from build123d import *

# Parameters (mm, degrees)
F0_W     = 250
F0_H     = 300
F0_W_2   = 105
F0_H_2   = 135
F1_DEPTH = 100
F3_DEPTH = 297


with BuildPart() as f1:
    # F0 (on Front) → F1 (new body)
    with BuildSketch(Plane.XZ):
        with Locations((62.479706, 83.388156)):
            Rectangle(F0_W, F0_H)
        with Locations((62.479706, 83.388156)):
            Rectangle(F0_W_2, F0_H_2, mode=Mode.SUBTRACT)
    extrude(amount=F1_DEPTH)

    # F2 (on face) → F3 (cut)
    with BuildSketch(Plane.YZ.offset(187.479706)):
        Polygon((-30.774537, -66.611844), (-100, 233.388156), (-100, -66.611844), align=None)
    extrude(amount=-F3_DEPTH, mode=Mode.SUBTRACT)


solid = f1.part
Work out the finished part from the listing and answer in its coordinate system (mm). A direction names the side the tool comes from. Give positions to 0.01 mm unless a question says otherwise; leave off trailing zeros. Loops run counter-clockwise (first coordinate to the right, second up) from the corner with the lowest first, then second, coordinate; pieces in that order, holes last. Notation, with made-up numbers: M -30,-12 L 21,-12 A26 cw 21,6 Z; hole C -37.75,9.25 d9. An arc over 180 degrees is marked long. Use CSV: the item, a comma, the result in double quotes.
1) Find section B-B on x = 26. Write down the section's boundary in (y, z), plus the area to 3 significant figures.
Answer:
outline,"M -100,233.39 L -80.96,150.89 L 0,150.89 L 0,233.39 Z; M -49.81,15.89 L -30.77,-66.61 L 0,-66.61 L 0,15.89 Z"
area,"10,800 mm^2"
2) Find section C-C on z = 94. Write down the section's boundary in (x, y), plus the area to 3 significant figures.
Answer:
outline,"M -62.52,-67.84 L 9.98,-67.84 L 9.98,0 L -62.52,0 Z; M 114.98,-67.84 L 187.48,-67.84 L 187.48,0 L 114.98,0 Z"
area,"9,840 mm^2"
3) Determine the mould class of faces 3 (the flat face through (-62.52, -38, 115)), 4 (the flat face through (119.785, -64.903, 81.288)), 5 (the flat face through (114.98, -31, 82)), 6 (the flat face through (62, -25, 15.888)) for opening direction X: released by +X, released by -X, zero draft, split by the parting line, or undercut.
Answer:
face 3,"released by -X"
face 4,"zero draft"
face 5,"undercut"
face 6,"undercut"
4) Find section A-A on y = -14.5. Write down the section's boundary in (x, z).
Answer:
outline,"M -62.52,-66.61 L 187.48,-66.61 L 187.48,233.39 L -62.52,233.39 Z; hole M 9.98,15.89 L 114.98,15.89 L 114.98,150.89 L 9.98,150.89 Z"
5) Consider L1, parallel to Z at x = 53.5, y = -5.5; L2, parallel to X at y = -28.5, z = 112.5; L3, parallel to Z at x = 99, y = -71. Determine where each line is inside the solid, lowest interval first.
Answer:
L1,"-66.61 to 15.89, 150.89 to 233.39"
L2,"-62.52 to 9.98, 114.98 to 187.48"
L3,"150.89 to 233.39"
6) Find section D-D on y = -38.5. Write down the section's boundary in (x, z), plus the area to 3 significant figures.
Answer:
outline,"M -62.52,-33.13 L 187.48,-33.13 L 187.48,233.39 L -62.52,233.39 Z; hole M 9.98,15.89 L 114.98,15.89 L 114.98,150.89 L 9.98,150.89 Z"
area,"52,500 mm^2"
7) Given P1, Ø12, axis at x = -8, z = 96.5, coming from the -Y side; P2, Ø1, axis at y = -50.5, z = 8.5, coming from the +X side; P3, Ø3, axis at x = 88.5, z = -13, coming from the -Y side, each flat-ended and moving along its own axis, determine where each tip first touches the part or whether it passes through.
Answer:
P1,"y = -69.8"
P2,"through"
P3,"y = -43.49"
8) Which of the six approach directions +Z, -Z, +X, -X, +Y, -Y give full straight-line access (tool end or side, diameter ignored) to faces 1 (the flat face through (9.98, -31, 82)), 2 (the flat face through (5, 0, 85))?
Answer:
face 1,"+Y, -Y"
face 2,"+Z, -Z, +X, -X, +Y"
